Can you work these out from the model? Positions are in its coordinate system, mm. A direction names the side the tool comes from. Coordinates: 2 decimals unless noted, no trailing zeros. Loops run counter-clockwise (first coordinate to the right, second up) from the corner with the lowest first, then second, coordinate; pieces in that order, holes last.
```python
from build123d import *

# Parameters (mm, degrees)
SKETCH1_R                = 120
BOSS_EXTRUDE1_DEPTH      = 10
SKETCH2_W                = 60
SKETCH2_H                = 40
BOSS_EXTRUDE2_DEPTH      = 10
CUT_EXTRUDE1_DEPTH       = 171.880074906
CUT_EXTRUDE1_DEPTH_BACK  = 171.880074906
SKETCH3_R                = 2.5
SKETCH4_R                = 5
BOSS_EXTRUDE4_DEPTH      = 10
SKETCH5_R                = 15
BOSS_EXTRUDE5_DEPTH      = 40
CUT_EXTRUDE2_DEPTH       = 179.222286063
CUT_EXTRUDE2_DEPTH_BACK  = 179.222286063
SKETCH7_R                = 10
SKETCH8_W                = 21
SKETCH8_H                = 21
BOSS_EXTRUDE8_DEPTH      = 20
BOSS_EXTRUDE9_DEPTH      = 42
BOSS_EXTRUDE9_DEPTH_BACK = 35.076669
SKETCH9_R                = 2.5


with BuildPart() as part:
    # Sketch1 → Boss-Extrude1 (new, symmetric)
    with BuildSketch(Plane(origin=(0, 0, 0), x_dir=(1, 0, 0), z_dir=(0, 1, 0))):
        with Locations(Location((0, 0, 0), (0, 0, 270))):
            Circle(SKETCH1_R)
    extrude(amount=BOSS_EXTRUDE1_DEPTH, both=True)

    # Sketch2 → Boss-Extrude2 (add)
    with BuildSketch(Plane(origin=(0, 10, 0), x_dir=(1, 0, 0), z_dir=(0, 1, 0))):
        with Locations((-80, 0)):
            Rectangle(SKETCH2_W, SKETCH2_H)
        with Locations((80, 0)):
            Rectangle(SKETCH2_W, SKETCH2_H)
    extrude(amount=BOSS_EXTRUDE2_DEPTH)

    # Sketch3 → Cut-Extrude1 (cut, two sides: drawn at the far end of the back side and taken through both)
    with BuildSketch(Plane(origin=(0, 10, 0), x_dir=(1, 0, 0), z_dir=(0, 1, 0)).offset(-CUT_EXTRUDE1_DEPTH_BACK)):
        with Locations(Location((0, 13, 0), (0, 0, 270))):
            Circle(SKETCH3_R)
    extrude(amount=CUT_EXTRUDE1_DEPTH + CUT_EXTRUDE1_DEPTH_BACK, mode=Mode.SUBTRACT)

    # Sketch4 → Boss-Extrude4 (add)
    with BuildSketch(Plane(origin=(-60, 0, 0), x_dir=(0, 0, -1), z_dir=(1, 0, 0))):
        with BuildLine():
            ThreePointArc((-20, 44.435128818), (0, 64.435128818), (20, 44.435128818))
            Line((20, 44.435128818), (20, 20))
            Line((20, 20), (-20, 20))
            Line((-20, 20), (-20, 44.435128818))
        make_face()
        with Locations((0, 40)):
            Circle(SKETCH4_R, mode=Mode.SUBTRACT)
    boss_extrude4 = extrude(amount=-BOSS_EXTRUDE4_DEPTH)

    # Sketch5 → Boss-Extrude5 (add)
    with BuildSketch(Plane.ZY.offset(70)):
        with BuildLine():
            Line((-20, 20), (20, 20))
            Line((20, 20), (20, 44.435128818))
            ThreePointArc((20, 44.435128818), (0, 64.435128818), (-20, 44.435128818))
            Line((-20, 44.435128818), (-20, 20))
        make_face()
        with Locations((0, 40)):
            Circle(SKETCH5_R, mode=Mode.SUBTRACT)
    extrude(amount=BOSS_EXTRUDE5_DEPTH)

    # Mirror2: Boss-Extrude4 across plane
    add(boss_extrude4.mirror(Plane(origin=(0, 0, 0), x_dir=(0, 0, 1), z_dir=(1, 0, 0))))

    # Sketch7 → Cut-Extrude2 (cut, two sides: drawn at the far end of the back side and taken through both)
    with BuildSketch(Plane(origin=(0, 10, 0), x_dir=(1, 0, 0), z_dir=(0, 1, 0)).offset(-CUT_EXTRUDE2_DEPTH_BACK)):
        with Locations(Location((0, 100, 0), (0, 0, 270))):
            Circle(SKETCH7_R)
        with Locations(Location((-70, -75, 0), (0, 0, 270))):
            Circle(SKETCH7_R)
        with Locations(Location((70, -75, 0), (0, 0, 270))):
            Circle(SKETCH7_R)
    extrude(amount=CUT_EXTRUDE2_DEPTH + CUT_EXTRUDE2_DEPTH_BACK, mode=Mode.SUBTRACT)

    # Sketch8 → Boss-Extrude8 (add)
    with BuildSketch(Plane(origin=(0, 10, 0), x_dir=(1, 0, 0), z_dir=(0, 1, 0))):
        with Locations((-70, -75)):
            Rectangle(SKETCH8_W, SKETCH8_H)
        with Locations((0, 100)):
            Rectangle(SKETCH8_W, SKETCH8_H)
        with Locations((70, -75)):
            Rectangle(SKETCH8_W, SKETCH8_H)
    extrude(amount=BOSS_EXTRUDE8_DEPTH)

    # Sketch9 → Boss-Extrude9 (add, two sides: drawn at the far end of the back side and taken through both)
    with BuildSketch(Plane(origin=(0, 0, 0), x_dir=(1, 0, 0), z_dir=(0, 1, 0)).offset(-BOSS_EXTRUDE9_DEPTH_BACK)):
        with Locations(Location((0, 12.5, 0), (0, 0, 270))):
            Circle(SKETCH9_R)
    extrude(amount=BOSS_EXTRUDE9_DEPTH + BOSS_EXTRUDE9_DEPTH_BACK)


solid = part.part
```
(1) I want a section at C-C on x = -5.5. Write out the boundary of the cut face in (y, z).
Check values:
outline: (-10, -119.87) - (10, -119.87) - (10, -110.5) - (30, -110.5) - (30, -89.5) - (10, -89.5) - (10, 119.87) - (-10, 119.87) - (-10, -91.65) - (10, -91.65) - (10, -108.35) - (-10, -108.35) - close
(2) Which directions (+Z, -Z, +X, -X, +Y, -Y) give clear straight access to the entire face, cutting with the end or side of a thin tool? Please do faces 4 (the flat face through (59.5, 20, 75)), 5 (the flat face through (0, 30, -100)), 6 (the flat face through (70, 10, 75)), 7 (the flat face through (60, 43, -5)).
Check values:
face 4: +Z, +Y
face 5: -Z, +X, -X, +Y
face 6: -Y
face 7: -Z, +Y
(3) I want a section at D-D on z = 75. Write out the boundary of the cut face in (x, y).
Check values:
outline: (-93.67, -10) - (-80, -10) - (-80, 10) - (-60, 10) - (-60, -10) - (60, -10) - (60, 10) - (80, 10) - (80, -10) - (93.67, -10) - (93.67, 10) - (80.5, 10) - (80.5, 30) - (59.5, 30) - (59.5, 10) - (-59.5, 10) - (-59.5, 30) - (-80.5, 30) - (-80.5, 10) - (-93.67, 10) - close
(4) I'm going to push flat-ended pins straight in: pin 1 (1.5 mm diameter, centred on x = -0.5, z = -12.5, fed in from +Y); pin 2 (16 mm diameter, centred on x = -3, y = 23.5, fed in from +Z); pin 3 (8 mm diameter, centred on y = 11.5, z = 69.5, fed in from -X). Where does each tip first touch, or does it pass through?
Check values:
pin 1: stops at y = 42
pin 2: stops at z = -10
pin 3: stops at x = -100.36
(5) If I drill on probe 1 along X at (y, z) = (28, -18.5); probe 2 along Y at (x, z) = (-93, 0); probe 3 along Y at (x, z) = (94, -19.5), over which ranges is the centre line in solid material (lowest first)?
Check values:
probe 1: x = -110 to -60, 60 to 70
probe 2: y = -10 to 25, 55 to 64.44
probe 3: y = -10 to 20
(6) If we mould it in two halves opening along Y, with no side actions, what happens to faces 1 (the flat face through (-86, 27, 20)), 2 (the flat face through (-70, 44, -4)), 3 (the flat face through (90, 20, 0))? For each: released by +Y, released by -Y, zero draft, split by the parting line, or undercut.
Check values:
face 1: zero draft
face 2: undercut
face 3: released by +Y
(7) I want a section at A-A on y = 16. Write out the boundary of the cut face in (x, z), then the cut area to 3 significant figures.
Check values:
outline: (-110, -20) - (-50, -20) - (-50, 20) - (-110, 20) - close; (-80.5, 64.5) - (-59.5, 64.5) - (-59.5, 85.5) - (-80.5, 85.5) - close; (-10.5, -110.5) - (10.5, -110.5) - (10.5, -89.5) - (-10.5, -89.5) - close; circle Ø5 at (0, -12.5); (50, -20) - (110, -20) - (110, 20) - (50, 20) - close; (59.5, 64.5) - (80.5, 64.5) - (80.5, 85.5) - (59.5, 85.5) - close
area: 6,140 mm2
(8) I want a section at B-B on z = 0. State how many separate pieces and enclosed holes the cut face has, then the cut area to 3 significant figures.
Check values:
separate pieces: 3
enclosed holes: 0
area: 7,270 mm2
